Source: CAD feature listing. Evaluate the final solid. Frame: model axes, mm. Face numbers are marked on the shaded views. A direction names the side the tool comes from. Round coordinates to 2 decimals unless told otherwise and drop trailing zeros. Loops run counter-clockwise (first coordinate to the right, second up) from the corner with the lowest first, then second, coordinate; pieces in that order, holes last. Notation, with made-up numbers: (78.5, 63.5) -> (95.5, 63.5) arc R13 cw to (95.5, 85.5) -> close; hole circle Ø1 at (79.25, -9). An arc over 180 degrees is marked (long way). Write item = value, one per line.
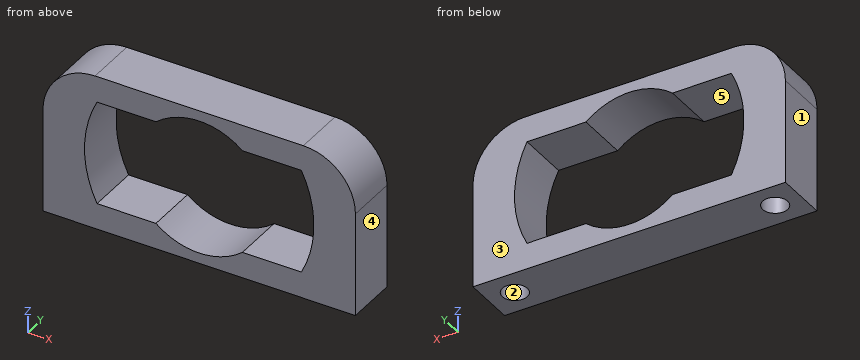
from build123d import *

# Parameters (mm, degrees)
SKETCH_1_W          = 60
SKETCH_1_H          = 30
EXTRUDE_1_DEPTH     = 10
FILLET_1_R          = 10
SKETCH_2_R          = 2.4
CUT_EXTRUDE_1_DEPTH = 6


with BuildPart() as part:
    # ｽｹｯﾁ1 → ﾎﾞｽ - 押し出し1 (new body)
    with BuildSketch(Plane(origin=(0, 0, 0), x_dir=(1, 0, 0), z_dir=(0, 1, 0))):
        Rectangle(SKETCH_1_W, SKETCH_1_H)
        with BuildLine():
            Line((19.629592456, -10), (8.306623863, -10))
            ThreePointArc((8.306623863, -10), (0, -13), (-8.306623863, -10))
            Line((-8.306623863, -10), (-19.629592456, -10))
            ThreePointArc((-19.629592456, -10), (-22.03, 0), (-19.629592456, 10))
            Line((-19.629592456, 10), (-8.306623863, 10))
            ThreePointArc((-8.306623863, 10), (0, 13), (8.306623863, 10))
            Line((8.306623863, 10), (19.629592456, 10))
            ThreePointArc((19.629592456, 10), (22.03, 0), (19.629592456, -10))
        make_face(mode=Mode.SUBTRACT)
    extrude(amount=EXTRUDE_1_DEPTH)

    # ﾌｨﾚｯﾄ1
    fillet_1_edges = [part.edges().sort_by_distance(p)[0] for p in [
        (30, 5, 15),
        (-30, 5, 15),
    ]]
    fillet(fillet_1_edges, radius=FILLET_1_R)

    # ｽｹｯﾁ2 → ｶｯﾄ - 押し出し1 (cut)
    with BuildSketch(Plane(origin=(0, 0, -15), x_dir=(-1, 0, 0), z_dir=(0, 0, -1))):
        with Locations((25, 5)):
            Circle(SKETCH_2_R)
        with Locations((-25, 5)):
            Circle(SKETCH_2_R)
    extrude(amount=-CUT_EXTRUDE_1_DEPTH, mode=Mode.SUBTRACT)


solid = part.part
1. Section query A-A (z = -11.25). Return the cut outline in (x, y), then the cut area to 3 significant figures.
Evaluation:
outline = (-30, 0) -> (-6.51, 0) -> (-6.51, 10) -> (-30, 10) -> close; (6.51, 0) -> (30, 0) -> (30, 10) -> (6.51, 10) -> close; hole circle Ø4.8 at (-25, 5); hole circle Ø4.8 at (25, 5)
area = 434 mm²
2. Section query C-C (y = 5). Return the cut outline in (x, z).
Evaluation:
outline = (-30, -15) -> (-27.4, -15) -> (-27.4, -9) -> (-22.6, -9) -> (-22.6, -15) -> (22.6, -15) -> (22.6, -9) -> (27.4, -9) -> (27.4, -15) -> (30, -15) -> (30, 5) arc R10 ccw to (20, 15) -> (-20, 15) arc R10 ccw to (-30, 5) -> close; hole (-19.63, -10) -> (-8.31, -10) arc R13 ccw to (8.31, -10) -> (19.63, -10) arc R22.03 ccw to (19.63, 10) -> (8.31, 10) arc R13 ccw to (-8.31, 10) -> (-19.63, 10) arc R22.03 ccw to start
3. Mould query, pull axis Y, two halves, no side actions, for the marked faces 1, 2 and 3. Classes: released by +Y, released by -Y, zero draft, split by the parting line, or undercut.
Evaluation:
face_1 = zero draft
face_2 = undercut
face_3 = released by +Y
4. Set-up query: the marked faces 4 and 5. Return all of +Z, -Z, +X, -X, +Y, -Y with unobstructed straight access to the full face (end or side cutting, diameter ignored); none if empty.
Evaluation:
face_4 = +Z, -Z, +X, +Y, -Y
face_5 = +Y, -Y
5. Section query B-B (x = -15). Return the cut outline in (y, z).
Evaluation:
outline = (0, -15) -> (10, -15) -> (10, -10) -> (0, -10) -> close; (0, 10) -> (10, 10) -> (10, 15) -> (0, 15) -> close
6. Line query: probe 1 along Y at (x, z) = (25, -13.6); probe 2 along Z at (x, y) = (-0.5, 2.75); probe 3 along Z at (x, y) = (12, 8). Output: solid intervals per line, ascending. Write a range as from..to.
Evaluation:
probe_1 = 0..2.6, 7.4..10
probe_2 = -15..-12.99, 12.99..15
probe_3 = -15..-10, 10..15
7. Contact query for flat-ended pins moving along their axis: pin 1 Ø3 at (x, y) = (-25, 5) entering from +Z; pin 2 Ø4 at (x, y) = (25, 5) entering from +Z; pin 3 Ø3 at (y, z) = (6.5, 10.5) entering from +X. Output: stop coordinate, or through.
Evaluation:
pin_1 = 14.37
pin_2 = 14.54
pin_3 = 29.17
8. Section query D-D (z = 0.5). Return the cut outline in (x, y), then the cut area to 3 significant figures.
Evaluation:
outline = (-30, 0) -> (-22.02, 0) -> (-22.02, 10) -> (-30, 10) -> close; (22.02, 0) -> (30, 0) -> (30, 10) -> (22.02, 10) -> close
area = 160 mm²
